For this review, take the finished solid that the model builds, in its own axes (mm). Round coordinates to 2 decimals unless told otherwise and drop trailing zeros. Order: outer loops, then holes, each group sorted by start corner. A loop starts at its lowest first (then second) coordinate and runs counter-clockwise, first axis right, second up. Notation, with made-up numbers: (-27.75, 88.25) - (10.25, 88.25) arc R21 cw to (10.25, 115.25) - close; hole circle Ø10 at (42.5, -37.75). An arc over 180 degrees is marked (long way). Write each question's results on one line, items separated by ' | '. Start each with the question number.
(1) For L1, parallel to Y at x = 2.8, z = 17.5 (3 decimals); L2, parallel to Z at x = 2.35, y = -41.5 (3 decimals); L3, parallel to Z at x = 0.8, y = -29.5 (3 decimals), list the stretches that pass through material, from the lowest coordinate up. Write a range as from..to.
(2) Take a section at C-C, the plane x = 1.05. Give the boundary of the cut face in (y, z) (3 decimals).
(3) Insertion check: pin 1 Ø1.6 at (x, z) = (1.5, 17.5) entering from +Y; pin 2 Ø2 at (y, z) = (-43, 7.5) entering from +X; pin 3 Ø1.6 at (x, y) = (1, 3) entering from -Z (3 decimals); pin 4 Ø1 at (x, z) = (1, 1) entering from -Y. Each pin has a flat end and moves straight along its axis. Give the tip position at first contact, or say it passes through.
(4) Take a section at D-D, the plane z = 1.75. Give the boundary of the cut face in (x, y) (3 decimals), plus the area to 3 significant figures.
(5) Take a section at B-B, the plane y = -39. Give the boundary of the cut face in (x, z) (3 decimals), plus the area to 3 significant figures.
(6) Take a section at A-A, the plane z = 14.5. Give the boundary of the cut face in (x, y) (3 decimals).
```python
from build123d import *

# Parameters (mm, degrees)
F1_DEPTH = 3.175


with BuildPart() as f1:
    # F0 (on Right) → F1 (new body)
    with BuildSketch(Plane.YZ):
        Polygon((-12.7, 0), (0, 0), (0, 3.175), (6.35, 3.175), (6.35, 9.525), (3.184586, 9.525), (3.184586, 22.225), (6.35, 22.225), (6.35, 28.575), (-69.85, 28.575), (-69.85, 25.4), (-69.85, 3.175), (-63.5, 3.175), (-63.5, 0), (-50.8, 0), (-50.8, 3.175), (-38.1, 3.175), (-38.1, 0), (-25.4, 0), (-25.4, 3.175), (-12.7, 3.175), align=None)
        Polygon((-66.675, 6.35), (-66.675, 25.4), (3.184586, 25.4), (0, 22.225), (0, 9.525), (3.184586, 6.35), align=None, mode=Mode.SUBTRACT)
    extrude(amount=F1_DEPTH)


solid = f1.part
```
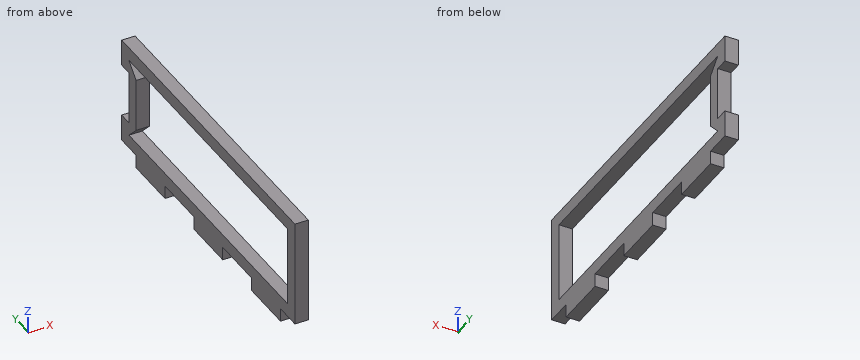
Results below:
1) L1: y = -69.85..-66.675, 0..3.185 | L2: z = 3.175..6.35, 25.4..28.575 | L3: z = 0..6.35, 25.4..28.575
2) outline: (-69.85, 3.175) - (-63.5, 3.175) - (-63.5, 0) - (-50.8, 0) - (-50.8, 3.175) - (-38.1, 3.175) - (-38.1, 0) - (-25.4, 0) - (-25.4, 3.175) - (-12.7, 3.175) - (-12.7, 0) - (0, 0) - (0, 3.175) - (6.35, 3.175) - (6.35, 9.525) - (3.185, 9.525) - (3.185, 22.225) - (6.35, 22.225) - (6.35, 28.575) - (-69.85, 28.575) - close; hole (-66.675, 6.35) - (3.185, 6.35) - (0, 9.525) - (0, 22.225) - (3.185, 25.4) - (-66.675, 25.4) - close
3) pin 1: stops at y = 3.18 | pin 2: passes through | pin 3: stops at z = 3.175 | pin 4: stops at y = -63.5
4) outline: (0, -63.5) - (3.175, -63.5) - (3.175, -50.8) - (0, -50.8) - close; (0, -38.1) - (3.175, -38.1) - (3.175, -25.4) - (0, -25.4) - close; (0, -12.7) - (3.175, -12.7) - (3.175, 0) - (0, 0) - close | area: 121 mm^2
5) outline: (0, 3.175) - (3.175, 3.175) - (3.175, 6.35) - (0, 6.35) - close; (0, 25.4) - (3.175, 25.4) - (3.175, 28.575) - (0, 28.575) - close | area: 20.2 mm^2
6) outline: (0, -69.85) - (3.175, -69.85) - (3.175, -66.675) - (0, -66.675) - close; (0, 0) - (3.175, 0) - (3.175, 3.185) - (0, 3.185) - close
